Input: part model. Units: mm. Frame: model coordinates. A direction names the side the tool comes from. Give positions to 0.01 mm unless a question says otherwise; leave off trailing zeros. Order: outer loops, then holes, each group sorted by start corner. A loop starts at its lowest first (then second) coordinate and runs counter-clockwise, first axis right, second up. Notation, with made-up numbers: (87.25, 3.25) - (126.25, 3.25) arc R24 cw to (126.25, 35.25) - close; hole circle Ø8 at (24.25, 30.25). An arc over 180 degrees is marked (long way). Use a Markdown table: item, result.
from build123d import *

# Parameters (mm, degrees)
BOSS_EXTRUDE1_DEPTH     = 2
SKETCH2_R               = 2.5
BOSS_EXTRUDE2_DEPTH     = 0.5
CUT_EXTRUDE1_DEPTH      = 40.182266397
CUT_EXTRUDE1_DEPTH_BACK = 40.182266397
SKETCH3_R               = 1.5
SKETCH3_R_2             = 1.3870402
SKETCH3_R_3             = 1.37388591
SKETCH3_R_4             = 1.428673318
SKETCH4_W               = 13.56544722
SKETCH4_H               = 12.948835983
BOSS_EXTRUDE3_DEPTH     = 2.3
SKETCH5_W               = 9.766151407
SKETCH5_H               = 11.19038182
BOSS_EXTRUDE4_DEPTH     = 2
SKETCH6_W               = 10
SKETCH6_H               = 7
BOSS_EXTRUDE5_DEPTH     = 4
SKETCH7_W               = 9.076584157
SKETCH7_H               = 3.089900989
SKETCH7_W_2             = 8.786905938
CUT_EXTRUDE2_DEPTH      = 5
SKETCH8_W               = 11.190381821
SKETCH8_H               = 9.155766944
BOSS_EXTRUDE6_DEPTH     = 3


with BuildPart() as part:
    # Sketch1 → Boss-Extrude1 (new body)
    with BuildSketch(Plane(origin=(0, 0, 0), x_dir=(1, 0, 0), z_dir=(0, 1, 0))):
        with BuildLine():
            Line((-31, 17.5), (31, 17.5))
            ThreePointArc((31, 17.5), (33.828427125, 16.328427125), (35, 13.5))
            Line((35, 13.5), (35, -13.5))
            ThreePointArc((35, -13.5), (33.828427125, -16.328427125), (31, -17.5))
            Line((31, -17.5), (-31, -17.5))
            ThreePointArc((-31, -17.5), (-33.828427125, -16.328427125), (-35, -13.5))
            Line((-35, -13.5), (-35, 13.5))
            ThreePointArc((-35, 13.5), (-33.828427125, 16.328427125), (-31, 17.5))
        make_face()
    extrude(amount=BOSS_EXTRUDE1_DEPTH)

    # Sketch2 → Boss-Extrude2 (add)
    with BuildSketch(Plane(origin=(0, 2, 0), x_dir=(1, 0, 0), z_dir=(0, 1, 0))):
        with Locations(Location((31.818181818, -14.393939394, 0), (0, 0, 270))):
            Circle(SKETCH2_R)
        with Locations(Location((-31.818181818, -14.393939394, 0), (0, 0, 270))):
            Circle(SKETCH2_R)
        with Locations(Location((-31.818181818, 14.393939394, 0), (0, 0, 270))):
            Circle(SKETCH2_R)
        with Locations(Location((31.818181818, 14.393939394, 0), (0, 0, 270))):
            Circle(SKETCH2_R)
    extrude(amount=BOSS_EXTRUDE2_DEPTH)

    # Sketch3 → Cut-Extrude1 (cut, two sides: drawn at the far end of the back side and taken through both)
    with BuildSketch(Plane(origin=(0, 2, 0), x_dir=(1, 0, 0), z_dir=(0, 1, 0)).offset(-CUT_EXTRUDE1_DEPTH_BACK)):
        with Locations(Location((31.818181818, -14.393939394, 0), (0, 0, 270))):
            Circle(SKETCH3_R)
        with Locations(Location((-31.818181818, -14.393939394, 0), (0, 0, 270))):
            Circle(SKETCH3_R_2)
        with Locations(Location((-31.818181818, 14.393939394, 0), (0, 0, 270))):
            Circle(SKETCH3_R_3)
        with Locations(Location((31.818181818, 14.393939394, 0), (0, 0, 270))):
            Circle(SKETCH3_R_4)
    extrude(amount=CUT_EXTRUDE1_DEPTH + CUT_EXTRUDE1_DEPTH_BACK, mode=Mode.SUBTRACT)

    # Sketch4 → Boss-Extrude3 (add)
    with BuildSketch(Plane(origin=(0, 2, 0), x_dir=(1, 0, 0), z_dir=(0, 1, 0))):
        with Locations((8.879537688, 1.123716819)):
            Rectangle(SKETCH4_W, SKETCH4_H)
    extrude(amount=BOSS_EXTRUDE3_DEPTH)

    # Sketch5 → Boss-Extrude4 (add)
    with BuildSketch(Plane(origin=(0, 2, 0), x_dir=(1, 0, 0), z_dir=(0, 1, 0))):
        with Locations((28.382877527, -2.187210992)):
            Rectangle(SKETCH5_W, SKETCH5_H)
    extrude(amount=BOSS_EXTRUDE4_DEPTH)

    # Sketch6 → Boss-Extrude5 (add)
    with BuildSketch(Plane(origin=(0, 2, 0), x_dir=(1, 0, 0), z_dir=(0, 1, 0))):
        with Locations((-9.446594787, 16)):
            Rectangle(SKETCH6_W, SKETCH6_H)
        with Locations((-23.101167125, 16)):
            Rectangle(SKETCH6_W, SKETCH6_H)
    extrude(amount=BOSS_EXTRUDE5_DEPTH)

    # Sketch7 → Cut-Extrude2 (cut)
    with BuildSketch(Plane(origin=(0, 0, -19.5), x_dir=(-1, 0, 0), z_dir=(0, 0, -1))):
        with Locations((9.33789674, 3.973358643)):
            Rectangle(SKETCH7_W, SKETCH7_H)
        with Locations((23.19417149, 3.973358643)):
            Rectangle(SKETCH7_W_2, SKETCH7_H)
    extrude(amount=-CUT_EXTRUDE2_DEPTH, mode=Mode.SUBTRACT)

    # Sketch8 → Boss-Extrude6 (add)
    with BuildSketch(Plane(origin=(0, 2, 0), x_dir=(1, 0, 0), z_dir=(0, 1, 0))):
        with Locations((19.328841327, 13.665477606)):
            Rectangle(SKETCH8_W, SKETCH8_H)
    extrude(amount=BOSS_EXTRUDE6_DEPTH)


solid = part.part
1. Section query C-C (z = 2.5). Return loops of the section in (x, y), then the cut area to 3 significant figures.
Response:
| item | result |
|---|---|
| outline | (-35, 0) - (35, 0) - (35, 2) - (33.27, 2) - (33.27, 4) - (23.5, 4) - (23.5, 2) - (15.66, 2) - (15.66, 4.3) - (2.1, 4.3) - (2.1, 2) - (-35, 2) - close |
| area | 191 mm^2 |
2. Section query B-B (y = 1.3). Return loops of the section in (x, z), then the cut area to 3 significant figures.
Response:
| item | result |
|---|---|
| outline | (-35, -13.5) arc R4 ccw to (-31, -17.5) - (31, -17.5) arc R4 ccw to (35, -13.5) - (35, 13.5) arc R4 ccw to (31, 17.5) - (-31, 17.5) arc R4 ccw to (-35, 13.5) - close; hole circle Ø2.77 at (-31.82, 14.39); hole circle Ø2.75 at (-31.82, -14.39); hole circle Ø3 at (31.82, 14.39); hole circle Ø2.86 at (31.82, -14.39) |
| area | 2,410 mm^2 |
3. Mould query, pull axis Y, two halves, no side actions, for faces 4 (the face through (-23, 2, -19)), 5 (the face through (-4.8, 4, -17)), 6 (the face through (-10, 4, -12.5)). Classes: pulls with the +Y half, pulls with the -Y half, needs draft (parallel to the pull), parting line crosses it, or undercut.
Response:
| item | result |
|---|---|
| face 4 | pulls with the -Y half |
| face 5 | undercut |
| face 6 | needs draft |
4. Pin query (flat end, axial travel): pin 1 (2.5 mm diameter, centred on y = 4, z = -14, fed in from -X); pin 2 (5 mm diameter, centred on x = 9, z = -4.5, fed in from +Y); pin 3 (3 mm diameter, centred on x = 18, y = 3, fed in from -Z). Return the tip coordinate at first contact, or that it passes through.
Response:
| item | result |
|---|---|
| pin 1 | stops at x = -28.1 |
| pin 2 | stops at y = 4.3 |
| pin 3 | stops at z = -18.24 |
5. Section query D-D (x = 3). Return loops of the section in (y, z), then the cut area to 3 significant figures.
Response:
| item | result |
|---|---|
| outline | (0, -17.5) - (2, -17.5) - (2, -7.6) - (4.3, -7.6) - (4.3, 5.35) - (2, 5.35) - (2, 17.5) - (0, 17.5) - close |
| area | 99.8 mm^2 |
6. Material intervals for line 1 along Y through (x, z) = (-7.5, -18); line 2 along X through (y, z) = (3.8, 4.5); line 3 along Y through (x, z) = (-20, -17), sorted ascending.
Response:
| item | result |
|---|---|
| line 1 | y = 2 to 2.43, 5.52 to 6 |
| line 2 | x = 2.1 to 15.66, 23.5 to 33.27 |
| line 3 | y = 0 to 2.43, 5.52 to 6 |
7. Section query A-A (x = 15). Return loops of the section in (y, z), then the cut area to 3 significant figures.
Response:
| item | result |
|---|---|
| outline | (0, -17.5) - (2, -17.5) - (2, -18.24) - (5, -18.24) - (5, -9.09) - (2, -9.09) - (2, -7.6) - (4.3, -7.6) - (4.3, 5.35) - (2, 5.35) - (2, 17.5) - (0, 17.5) - close |
| area | 127 mm^2 |
8. Set-up query: faces 1 (the face through (-18.101, 4, -16)), 2 (the face through (31, 2.5, -13)), 3 (the face through (33.926, 2.246, -13.05)). Return all of +Z, -Z, +X, -X, +Y, -Y with unobstructed straight access to the full face (end or side cutting, diameter ignored); none if empty.
Response:
| item | result |
|---|---|
| face 1 | +Z, -Z, +Y |
| face 2 | -Z, +X, +Y |
| face 3 | +Y |
